from build123d import *

# Parameters (mm, degrees)
SKETCH1_W           = 51
SKETCH1_H           = 18.5
BOSS_EXTRUDE1_DEPTH = 1.5
SKETCH2_W           = 32
SKETCH2_H           = 11.5
BOSS_EXTRUDE2_DEPTH = 1.5
SKETCH3_W           = 5
SKETCH3_H           = 7.7
BOSS_EXTRUDE3_DEPTH = 2.5
SKETCH4_W           = 4.3
SKETCH4_H           = 7.5
BOSS_EXTRUDE4_DEPTH = 4
SKETCH5_W           = 25
SKETCH5_H           = 8.65
CUT_EXTRUDE1_DEPTH  = 0.01


with BuildPart() as part:
    # Sketch1 → Boss-Extrude1 (new body)
    with BuildSketch(Plane(origin=(0, 0, 27), x_dir=(1, 0, 0), z_dir=(0, 1, 0))):
        with Locations((25.5, 27)):
            Rectangle(SKETCH1_W, SKETCH1_H)
    extrude(amount=BOSS_EXTRUDE1_DEPTH)

    # Sketch2 → Boss-Extrude2 (add)
    with BuildSketch(Plane(origin=(0, 1.5, 0), x_dir=(1, 0, 0), z_dir=(0, 1, 0))):
        with Locations((21, 0)):
            Rectangle(SKETCH2_W, SKETCH2_H)
    extrude(amount=BOSS_EXTRUDE2_DEPTH)

    # Sketch3 → Boss-Extrude3 (add)
    with BuildSketch(Plane(origin=(0, 1.5, 0), x_dir=(1, 0, 0), z_dir=(0, 1, 0))):
        with Locations((48.5, 0)):
            Rectangle(SKETCH3_W, SKETCH3_H)
    extrude(amount=BOSS_EXTRUDE3_DEPTH)

    # Sketch4 → Boss-Extrude4 (add)
    with BuildSketch(Plane.XZ):
        with Locations((46.85, 0)):
            Rectangle(SKETCH4_W, SKETCH4_H)
    extrude(amount=BOSS_EXTRUDE4_DEPTH)

    # Sketch5 → Cut-Extrude1 (cut)
    with BuildSketch(Plane(origin=(0, 3, 0), x_dir=(1, 0, 0), z_dir=(0, 1, 0))):
        with Locations((24, -1.025)):
            Rectangle(SKETCH5_W, SKETCH5_H)
    extrude(amount=-CUT_EXTRUDE1_DEPTH, mode=Mode.SUBTRACT)


solid = part.part
The listing builds one solid part. Answer for the finished solid, in the listing's coordinates (mm). A direction names the side the tool comes from. Give positions to 0.01 mm unless a question says otherwise; leave off trailing zeros. Order: outer loops, then holes, each group sorted by start corner. A loop starts at its lowest first (then second) coordinate and runs counter-clockwise, first axis right, second up. Notation, with made-up numbers: (88, 74) - (124, 74) arc R5 ccw to (124, 80) - close; hole circle Ø8 at (-20.75, 50.5). An arc over 180 degrees is marked (long way). Use one line per item in the form item = value.
1) Find section B-B on x = 6. Determine the outline of the cut face in (y, z), and give its area (3 significant figures).
Verdict:
outline = (0, -9.25) - (1.5, -9.25) - (1.5, -5.75) - (3, -5.75) - (3, 5.75) - (1.5, 5.75) - (1.5, 9.25) - (0, 9.25) - close
area = 45.0 mm^2
2) For faces 1 (the flat face through (47, -2, -3.75)), 2 (the flat face through (21, 2, 5.75)), 3 (the flat face through (44.7, -2, 0)), 4 (the flat face through (14, 3, -4)), determine the directions among +Z, -Z, +X, -X, +Y, -Y from which every point of the face is accessible in a straight line to the end or side of a thin tool.
Verdict:
face_1 = -Z, +X, -X, -Y
face_2 = +Z, +X, -X, +Y
face_3 = +Z, -Z, -X, -Y
face_4 = +Z, -Z, -X, +Y
3) Each of these flat-tipped pins is pushed along its axis until it touches: pin 1 (4.5 mm diameter, centred on x = 46.5, y = -3, fed in from -Z); pin 2 (1.2 mm diameter, centred on x = 19.5, y = 2.5, fed in from -Z); pin 3 (4 mm diameter, centred on x = 23.5, z = 4.5, fed in from -Y). Where does it stop, or does it pass through?
Verdict:
pin_1 = -3.75
pin_2 = -5.75
pin_3 = 0
4) The mould has two halves that part along X. Classify faces 5 (the flat face through (48, 3, -3.85)), 6 (the flat face through (51, 2, 0)), 7 (the flat face through (37, 2, 0)): released by +X, released by -X, zero draft, split by the parting line, or undercut.
Verdict:
face_5 = zero draft
face_6 = released by +X
face_7 = undercut
5) Find section A-A on y = 2.5. Determine the outline of the cut face in (x, z).
Verdict:
outline = (5, -5.75) - (37, -5.75) - (37, 5.75) - (5, 5.75) - close; (46, -3.85) - (51, -3.85) - (51, 3.85) - (46, 3.85) - close
6) Consider probe 1 along Y at (x, z) = (13, -7.25); probe 2 along X at (y, z) = (-0.5, -1.5); probe 3 along Z at (x, y) = (17, 1.75). Determine where each line is inside the solid, lowest interval first. Write a range as [from, to].
Verdict:
probe_1 = [0, 1.5]
probe_2 = [44.7, 49]
probe_3 = [-5.75, 5.75]
